from build123d import *

# Parameters (mm, degrees)
SKETCH1_R           = 2.75
BOSS_EXTRUDE1_DEPTH = 3.175


with BuildPart() as part:
    # Sketch1 → Boss-Extrude1 (new body)
    with BuildSketch(Plane.XY):
        with BuildLine():
            Line((-94.828483368, -355.15), (-204.828483368, -355.15))
            Line((-204.828483368, -355.15), (-209.932915484, -336.1))
            Line((-209.932915484, -336.1), (-155.261017178, -336.1))
            ThreePointArc((-155.261017178, -336.1), (-145.615191064, -338.971618374), (-135.96936495, -336.1))
            Line((-135.96936495, -336.1), (-94.828483368, -336.1))
            Line((-94.828483368, -336.1), (-94.828483368, -355.15))
        make_face()
        with Locations((-121.828483368, -343.6)):
            Circle(SKETCH1_R, mode=Mode.SUBTRACT)
        with Locations((-172.748438952, -343.6)):
            Circle(SKETCH1_R, mode=Mode.SUBTRACT)
    extrude(amount=-BOSS_EXTRUDE1_DEPTH)


solid = part.part
Check sheet for the modelled part. Datum: model origin and axes. Units: mm. Round coordinates to 2 decimals unless told otherwise and drop trailing zeros. Loops run counter-clockwise (first coordinate to the right, second up) from the corner with the lowest first, then second, coordinate; pieces in that order, holes last.
1. Sectioned sample at C-C on y = -350.25. Record the boundary of the cut face in (x, z) (3 decimals), and give its area (3 significant figures).
2. Sectioned sample at A-A on z = -0.6. Record the boundary of the cut face in (x, y).
3. Scan lines: probe 1 along X at (y, z) = (-343.6, -1.1); probe 2 along X at (y, z) = (-345.5, -2.35); probe 3 along Y at (x, z) = (-172, -2.6). Record each from-to range of solid material in increasing order.
4. Mould release check, pull along X, two halves, no side actions. Record for faces 1 (the flat face through (-207.345, -345.758, -1.565)), 2 (the cylindrical face through (-120.56, -346.04, -1.57)), 3 (the flat face through (-152, -345, 0)): released by +X, released by -X, zero draft, split by the parting line, or undercut.
5. Sectioned sample at B-B on y = -343.6. Record the boundary of the cut face in (x, z) (3 decimals), and give its area (3 significant figures).
Recorded:
1. outline: (-206.141, -3.175) - (-94.828, -3.175) - (-94.828, 0) - (-206.141, 0) - close
1. area: 353 mm2
2. outline: (-209.93, -336.1) - (-204.83, -355.15) - (-94.83, -355.15) - (-94.83, -336.1) - (-135.97, -336.1) arc R17.64 cw to (-155.26, -336.1) - close; hole circle Ø5.5 at (-172.75, -343.6); hole circle Ø5.5 at (-121.83, -343.6)
3. probe 1: x = -207.92 to -175.5, -170 to -124.58, -119.08 to -94.83
3. probe 2: x = -207.41 to -174.74, -170.76 to -123.82, -119.84 to -94.83
3. probe 3: y = -355.15 to -346.25, -340.95 to -336.1
4. face 1: released by -X
4. face 2: undercut
4. face 3: zero draft
5. outline: (-207.923, -3.175) - (-175.498, -3.175) - (-175.498, 0) - (-207.923, 0) - close; (-169.998, -3.175) - (-124.578, -3.175) - (-124.578, 0) - (-169.998, 0) - close; (-119.078, -3.175) - (-94.828, -3.175) - (-94.828, 0) - (-119.078, 0) - close
5. area: 324 mm2
